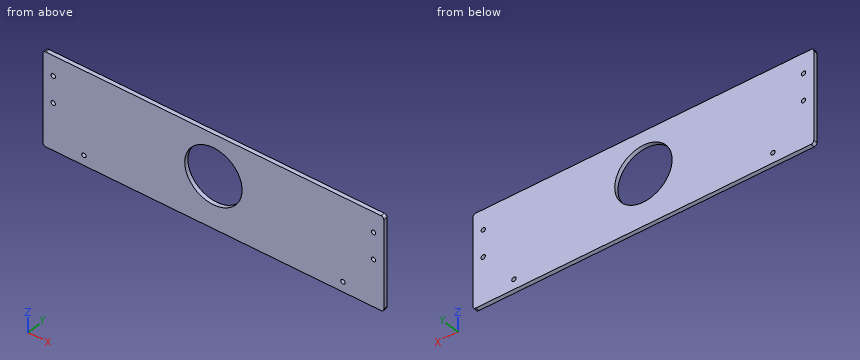
from build123d import *

# Parameters (mm, degrees)
SKETCH_1_W          = 250
SKETCH_1_H          = 70
EXTRUDE_1_DEPTH     = 3
SKETCH_2_R          = 1.6
CUT_EXTRUDE_1_DEPTH = 130.842211934
FILLET_2_R          = 2
SKETCH_3_R          = 21.05
CUT_EXTRUDE_2_DEPTH = 130.842211934


with BuildPart() as part:
    # 草图1 → 凸台-拉伸1 (new body)
    with BuildSketch(Plane(origin=(0, 0, 0), x_dir=(1, 0, 0), z_dir=(0, 1, 0))):
        Rectangle(SKETCH_1_W, SKETCH_1_H)
    extrude(amount=EXTRUDE_1_DEPTH)

    # 草图2 → 切除-拉伸1 (cut, through all)
    with BuildSketch(Plane(origin=(0, 3, 0), x_dir=(1, 0, 0), z_dir=(0, 1, 0))):
        with Locations(Location((-95, 27.5, 0), (0, 0, 270))):
            Circle(SKETCH_2_R)
        with Locations(Location((95, 27.5, 0), (0, 0, 270))):
            Circle(SKETCH_2_R)
        with Locations(Location((-117.5, 0, 0), (0, 0, 270))):
            Circle(SKETCH_2_R)
        with Locations(Location((-117.5, -20, 0), (0, 0, 270))):
            Circle(SKETCH_2_R)
        with Locations(Location((117.5, -20, 0), (0, 0, 90))):
            Circle(SKETCH_2_R)
        with Locations(Location((117.5, 0, 0), (0, 0, 90))):
            Circle(SKETCH_2_R)
    extrude(amount=-CUT_EXTRUDE_1_DEPTH, mode=Mode.SUBTRACT)

    # 圆角2
    fillet_2_edges = [part.edges().sort_by_distance(p)[0] for p in [
        (125, 1.5, 35),
        (-125, 1.5, 35),
        (-125, 1.5, -35),
        (125, 1.5, -35),
    ]]
    fillet(fillet_2_edges, radius=FILLET_2_R)

    # 草图3 → 切除-拉伸2 (cut, through all)
    with BuildSketch(Plane(origin=(0, 3, 0), x_dir=(1, 0, 0), z_dir=(0, 1, 0))):
        with Locations(Location((0, -3.75, 0), (0, 0, 270))):
            Circle(SKETCH_3_R)
    extrude(amount=-CUT_EXTRUDE_2_DEPTH, mode=Mode.SUBTRACT)


solid = part.part
Geometry check sheet. Reference: the model listing, model coordinates, mm. Give positions to 0.01 mm unless a question says otherwise; leave off trailing zeros. Loops run counter-clockwise (first coordinate to the right, second up) from the corner with the lowest first, then second, coordinate; pieces in that order, holes last. Notation, with made-up numbers: M -25.5,61 L -6.5,61 A22 ccw -6.5,84 Z; hole C 70.5,77.25 d9. An arc over 180 degrees is marked long. Write each question's results on one line, items separated by ' | '.
1) Section check A-A, the plane y = 0.85. Record the boundary of the cut face in (x, z), plus the area to 3 significant figures.
Answers follow:
outline: M -125,-33 A2 ccw -123,-35 L 123,-35 A2 ccw 125,-33 L 125,33 A2 ccw 123,35 L -123,35 A2 ccw -125,33 Z; hole C -117.5,0 d3.2; hole C -117.5,20 d3.2; hole C -95,-27.5 d3.2; hole C 0,3.75 d42.1; hole C 95,-27.5 d3.2; hole C 117.5,0 d3.2; hole C 117.5,20 d3.2 | area: 16,100 mm2
2) Thickness scan on line 1 (Z direction, x = 117.5, y = 2.2); line 2 (Z direction, x = -95, y = 1.25); line 3 (X direction, y = 0.4, z = 20). Record the ranges inside material, lowest first.
Answers follow:
line 1: -35 to -1.6, 1.6 to 18.4, 21.6 to 35 | line 2: -35 to -29.1, -25.9 to 35 | line 3: -125 to -119.1, -115.9 to -13.38, 13.38 to 115.9, 119.1 to 125
3) Section check C-C, the plane z = -12. Record the boundary of the cut face in (x, y).
Answers follow:
outline: M -125,0 L -13.97,0 L -13.97,3 L -125,3 Z; M 13.97,0 L 125,0 L 125,3 L 13.97,3 Z
4) Section check B-B, the plane z = 15.5. Record the boundary of the cut face in (x, y).
Answers follow:
outline: M -125,0 L -17.47,0 L -17.47,3 L -125,3 Z; M 17.47,0 L 125,0 L 125,3 L 17.47,3 Z
